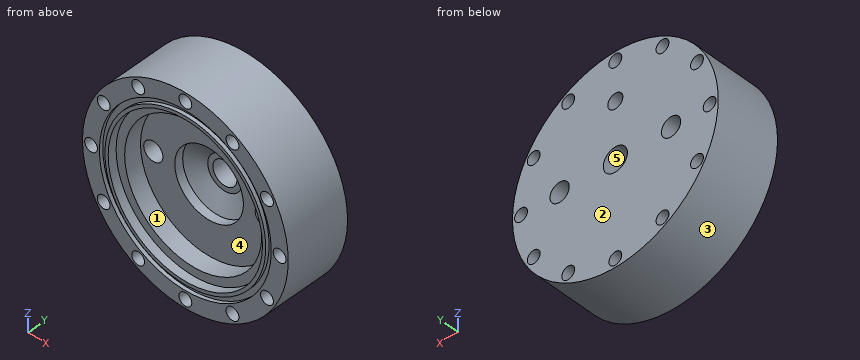
```python
from build123d import *

# Parameters (mm, degrees)
CIRPATTERN1_COUNT                 = 12
PIPE_TAP_DRILL_FOR_1_2_TAP1_D     = 17.8562
PIPE_TAP_DRILL_FOR_1_2_TAP1_DEPTH = 19.05
PIPE_TAP_DRILL_FOR_1_2_TAP1_TIP   = 5.364543693
CIRPATTERN2_COUNT                 = 2
PIPE_TAP_DRILL_FOR_1_4_TAP1_D     = 11.1252
PIPE_TAP_DRILL_FOR_1_4_TAP1_DEPTH = 31.75
PIPE_TAP_DRILL_FOR_1_4_TAP1_TIP   = 3.342347279


with BuildPart() as part:
    # Sketch1 → Revolve1 (revolve)
    with BuildSketch(Plane.XY):
        Polygon((0, 0), (-76.2, 0), (-76.2, -47.6377), (-63.6524, -47.6377), (-63.6524, -44.9453), (-59.5884, -44.9453), (-59.5884, -47.6377), (-57.15, -47.6377), (-57.15, -41.2877), (-50.8, -41.2877), (-50.8, -28.5877), (-25.4, -28.5877), (-25.4, -22.2377), (-12.7, -15.8877), (0, -15.8877), align=None)
    revolve(axis=Axis((0, -15.8877, 0), (0, 1, 0)))

    # Sketch3 → 3/8 (0.375) Diameter Hole1 (revolve, cut)
    with BuildSketch(Plane(origin=(-69.85, 0, 0), x_dir=(0, 0, 1), z_dir=(1, 0, 0))):
        Polygon((0, 0), (0, 60.011598698), (4.7625, 57.15), (4.7625, 0), align=None)
    f_3_8_0_375_diameter_hole1 = revolve(axis=Axis((-69.85, 6.35, 0), (0, -1, 0)), mode=Mode.SUBTRACT)

    # CirPattern1: 3/8 (0.375) Diameter Hole1 ×12 about axis
    cirpattern1_axis = Axis((0, 0, 0), (0, 1, 0))
    for i in range(1, CIRPATTERN1_COUNT):
        add(f_3_8_0_375_diameter_hole1.rotate(cirpattern1_axis, i * 360 / CIRPATTERN1_COUNT), mode=Mode.SUBTRACT)

    # Pipe Tap Drill for 1/2 Tap1
    with Locations(Plane(origin=(0, 0, 0), x_dir=(1, 0, 0), z_dir=(0, 1, 0))):
        with Locations((0, 0)):
            Hole(PIPE_TAP_DRILL_FOR_1_2_TAP1_D / 2, depth=PIPE_TAP_DRILL_FOR_1_2_TAP1_DEPTH)
            with Locations((0, 0, -(PIPE_TAP_DRILL_FOR_1_2_TAP1_DEPTH + PIPE_TAP_DRILL_FOR_1_2_TAP1_TIP / 2))):  # 118° drill point
                Cone(0, PIPE_TAP_DRILL_FOR_1_2_TAP1_D / 2, PIPE_TAP_DRILL_FOR_1_2_TAP1_TIP, mode=Mode.SUBTRACT)

    # Sketch7 → Pipe Tap Drill for 3/8 Tap1 (revolve, cut)
    with BuildSketch(Plane(origin=(-41.275, 0, 0), x_dir=(0, 0, 1), z_dir=(1, 0, 0))):
        Polygon((0, 0), (0, 36.038582582), (7.1374, 31.75), (7.1374, 0), align=None)
    pipe_tap_drill_for_3_8_tap1 = revolve(axis=Axis((-41.275, 6.35, 0), (0, -1, 0)), mode=Mode.SUBTRACT)

    # CirPattern2: Pipe Tap Drill for 3/8 Tap1 ×2 about axis
    cirpattern2_axis = Axis((0, 0, 0), (0, 1, 0))
    for i in range(1, CIRPATTERN2_COUNT):
        add(pipe_tap_drill_for_3_8_tap1.rotate(cirpattern2_axis, i * 360 / CIRPATTERN2_COUNT), mode=Mode.SUBTRACT)

    # Pipe Tap Drill for 1/4 Tap1
    with Locations(Plane(origin=(0, 0, 0), x_dir=(1, 0, 0), z_dir=(0, 1, 0))):
        with Locations((0, -41.275)):
            Hole(PIPE_TAP_DRILL_FOR_1_4_TAP1_D / 2, depth=PIPE_TAP_DRILL_FOR_1_4_TAP1_DEPTH)
            with Locations((0, 0, -(PIPE_TAP_DRILL_FOR_1_4_TAP1_DEPTH + PIPE_TAP_DRILL_FOR_1_4_TAP1_TIP / 2))):  # 118° drill point
                Cone(0, PIPE_TAP_DRILL_FOR_1_4_TAP1_D / 2, PIPE_TAP_DRILL_FOR_1_4_TAP1_TIP, mode=Mode.SUBTRACT)


solid = part.part
```
Verification items for the finished model (mm, model axes). Face numbers are marked on the shaded views. A direction names the side the tool comes from. Round coordinates to 2 decimals unless told otherwise and drop trailing zeros. Order: outer loops, then holes, each group sorted by start corner. A loop starts at its lowest first (then second) coordinate and runs counter-clockwise, first axis right, second up. Notation, with made-up numbers: (44.5, 24) - (91.5, 24) arc R27 ccw to (91.5, 58) - close; hole circle Ø7 at (58.5, 48). An arc over 180 degrees is marked (long way). Use CSV: the item, a comma, the result in double quotes. Start each with the question number.
1) Mould release check, pull along X, two halves, no side actions. Record for the marked faces 1, 2 and 3: +X half, -X half, draft (parallel to the pull), parting line (faces both ways), or undercut.
2) Access from +Z, -Z, +X, -X, +Y, -Y to the whole of each face (thin tool, end or side, straight path). Record for the marked faces 4 and 5.
3) Section check A-A, the plane x = -69.85. Record the cut outline in (y, z), plus the area to 3 significant figures.
4) Section check B-B, the plane y = -3.5. State how many separate pieces and enclosed holes the cut face has, plus the area to 3 significant figures.
5) Section check C-C, the plane z = 69.85. Record the cut outline in (x, y), plus the area to 3 significant figures.
6) Thickness scan on L1, parallel to X at y = -2, z = -4; L2, parallel to X at y = -28, z = 6.5; L3, parallel to Z at x = -63, y = -19. Record the ranges inside material, lowest first.
7) Go/stop test with flat-tipped pins: P1, Ø3, axis at x = 4.5, y = -9.5, coming from the +Z side; P2, Ø1, axis at x = 47, y = -6.5, coming from the -Z side; P3, Ø4, axis at x = -11, y = -41.5, coming from the +Z side. Record where each tip stops, or that it passes through.
Answers:
1,face 1,"undercut"
1,face 2,"draft"
1,face 3,"parting line"
2,face 4,"-Y"
2,face 5,"+Y, -Y"
3,outline,"(-47.64, -30.45) - (0, -30.45) - (0, -4.76) - (-47.64, -4.76) - close; (-47.64, 4.76) - (0, 4.76) - (0, 30.45) - (-47.64, 30.45) - close"
3,area,"2,450 mm²"
4,separate pieces,"1"
4,enclosed holes,"16"
4,area,"16,700 mm²"
5,outline,"(-30.45, -47.64) - (-4.76, -47.64) - (-4.76, 0) - (-30.45, 0) - close; (4.76, -47.64) - (30.45, -47.64) - (30.45, 0) - (4.76, 0) - close"
5,area,"2,450 mm²"
6,L1,"x = -76.09 to -72.43, -67.27 to -47.19, -35.36 to -7.98, 7.98 to 35.36, 47.19 to 67.27, 72.43 to 76.09"
6,L2,"x = -75.92 to -44.22, -38.33 to -24.55, 24.55 to 38.33, 44.22 to 75.92"
6,L3,"z = -42.87 to -38.97, -30.88 to 30.88, 38.97 to 42.87"
7,P1,"stops at z = 76.14"
7,P2,"stops at z = -60.37"
7,P3,"stops at z = 75.67"
